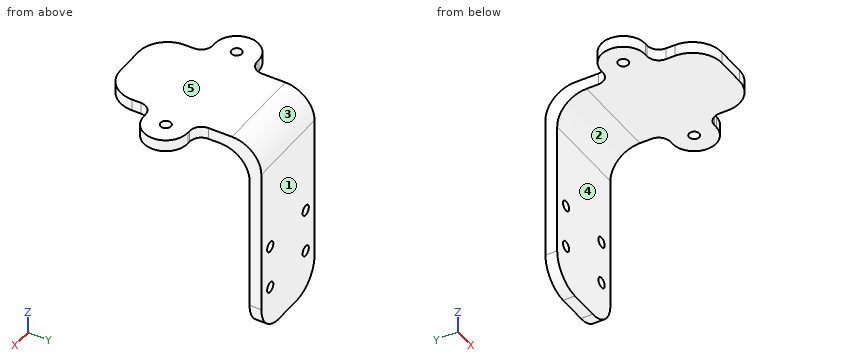
from build123d import *

# Parameters (mm, degrees)
SKETCH1_W            = 30
SKETCH1_H            = 70
BOSS_EXTRUDE1_DEPTH  = 2
SKETCH2_W            = 30
SKETCH2_H            = 4
BOSS_EXTRUDE2_DEPTH  = 50
SKETCH3_R            = 1.75
BOSS_EXTRUDE3_DEPTH  = 4
SKETCH4_R            = 1.75
CUT_EXTRUDE1_DEPTH   = 4
LPATTERN1_COUNT      = 2
LPATTERN1_PITCH      = 15
LPATTERN1_COUNT_DIR2 = 2
LPATTERN1_PITCH_DIR2 = 20
FILLET1_R            = 10
FILLET2_R            = 4


with BuildPart() as part:
    # Sketch1 → Boss-Extrude1 (new body, symmetric)
    with BuildSketch(Plane(origin=(0, 0, 0), x_dir=(1, 0, 0), z_dir=(0, 1, 0))):
        Rectangle(SKETCH1_W, SKETCH1_H)
    extrude(amount=BOSS_EXTRUDE1_DEPTH, both=True)

    # Sketch2 → Boss-Extrude2 (add)
    with BuildSketch(Plane.XZ.offset(2)):
        with Locations((0, 33)):
            Rectangle(SKETCH2_W, SKETCH2_H)
    extrude(amount=BOSS_EXTRUDE2_DEPTH)

    # Sketch3 → Boss-Extrude3 (add)
    with BuildSketch(Plane.XY.offset(35)):
        with BuildLine():
            Line((20, -20), (-20, -20))
            ThreePointArc((-20, -20), (-27.5, -27.5), (-20, -35))
            Line((-20, -35), (20, -35))
            ThreePointArc((20, -35), (27.5, -27.5), (20, -20))
        make_face()
        with Locations((-20, -27.5)):
            Circle(SKETCH3_R, mode=Mode.SUBTRACT)
        with Locations((20, -27.5)):
            Circle(SKETCH3_R, mode=Mode.SUBTRACT)
    extrude(amount=-BOSS_EXTRUDE3_DEPTH)

    # Sketch4 → Cut-Extrude1 (cut)
    with BuildSketch(Plane(origin=(0, 2, 0), x_dir=(1, 0, 0), z_dir=(0, 1, 0))):
        with Locations((-10, 20)):
            Circle(SKETCH4_R)
    cut_extrude1 = extrude(amount=-CUT_EXTRUDE1_DEPTH, mode=Mode.SUBTRACT)

    # LPattern1: Cut-Extrude1 2 × 2
    with Locations(*[(j * LPATTERN1_PITCH_DIR2, 0, i * LPATTERN1_PITCH) for i in range(LPATTERN1_COUNT) for j in range(LPATTERN1_COUNT_DIR2) if (i, j) != (0, 0)]):
        add(cut_extrude1, mode=Mode.SUBTRACT)

    # Fillet1
    fillet1_edges = [part.edges().sort_by_distance(p)[0] for p in [
        (0, -2, 31),
        (15, -52, 33),
        (0, 2, 35),
        (-15, -52, 33),
        (-15, 0, -35),
        (15, 0, -35),
    ]]
    fillet(fillet1_edges, radius=FILLET1_R)

    # Fillet2
    fillet2_edges = [part.edges().sort_by_distance(p)[0] for p in [
        (15, -35, 33),
        (-15, -35, 33),
        (15, -20, 33),
        (-15, -20, 33),
    ]]
    fillet(fillet2_edges, radius=FILLET2_R)


solid = part.part
Work out the finished part from the listing and answer in its coordinate system (mm). Face numbers are marked on the shaded views. A direction names the side the tool comes from. Give positions to 0.01 mm unless a question says otherwise; leave off trailing zeros. Loops run counter-clockwise (first coordinate to the right, second up) from the corner with the lowest first, then second, coordinate; pieces in that order, holes last. Notation, with made-up numbers: (45, -21.5) -> (65, -21.5) arc R32 ccw to (65, 9.5) -> close; hole circle Ø7 at (-34.75, 49.5). An arc over 180 degrees is marked (long way). Use a Markdown table: item, result. Add a question column.
1) Each of these flat-tipped pins is pushed along its axis until it touches: P1, Ø5, axis at x = 0, y = -25.5, coming from the -Z side; P2, Ø20, axis at y = -10.5, z = 3.5, coming from the +X side; P3, Ø1.1, axis at x = 19.5, z = 34, coming from the -Y side; P4, Ø6, axis at x = -17, z = 25, coming from the +Y side. Where does it stop, or does it pass through?
2) For a pull along Z with two mould halves and no side action, classify the marked faces 1, 2 and 3 as +Z half, -Z half, draft (parallel to the pull), parting line (faces both ways), or undercut.
3) The part is cut by section A-A, the plane y = -27.5. Determine the outline of the cut face in (x, z).
4) Which of the six approach directions +Z, -Z, +X, -X, +Y, -Y give full straight-line access (tool end or side, diameter ignored) to the marked faces 4 and 5?
5) The part is cut by section D-D, the plane x = -0.5. Determine the outline of the cut face in (y, z), plus the area to 3 significant figures.
6) The part is cut by section B-B, the plane z = -20. Determine the outline of the cut face in (x, y), plus the area to 3 significant figures.
7) Consider line 1 along X through (y, z) = (0, -5); line 2 along Z through (x, y) = (-10, 0); line 3 along Z through (x, y) = (-10, -0.85). Determine where each line is inside the solid, lowest interval first.
8) The part is cut by section C-C, the plane x = 10. Determine the outline of the cut face in (y, z), plus the area to 3 significant figures.
Reported:
| question | item | result |
|---|---|---|
| 1 | P1 | stops at z = 31 |
| 1 | P2 | stops at x = 15 |
| 1 | P3 | stops at y = -35 |
| 1 | P4 | stops at y = 2 |
| 2 | face 1 | draft |
| 2 | face 2 | -Z half |
| 2 | face 3 | +Z half |
| 3 | outline | (-27.5, 31) -> (-21.75, 31) -> (-21.75, 35) -> (-27.5, 35) -> close; (-18.25, 31) -> (18.25, 31) -> (18.25, 35) -> (-18.25, 35) -> close; (21.75, 31) -> (27.5, 31) -> (27.5, 35) -> (21.75, 35) -> close |
| 4 | face 4 | -Z, +X, -X, -Y |
| 4 | face 5 | +Z, +X, -X, +Y, -Y |
| 5 | outline | (-52, 31) -> (-12, 31) arc R10 cw to (-2, 21) -> (-2, -35) -> (2, -35) -> (2, 25) arc R10 ccw to (-8, 35) -> (-52, 35) -> close |
| 5 | area | 480 mm^2 |
| 6 | outline | (-15, -2) -> (-11.75, -2) -> (-11.75, 2) -> (-15, 2) -> close; (-8.25, -2) -> (8.25, -2) -> (8.25, 2) -> (-8.25, 2) -> close; (11.75, -2) -> (15, -2) -> (15, 2) -> (11.75, 2) -> close |
| 6 | area | 92.0 mm^2 |
| 7 | line 1 | x = -15 to -11.75, -8.25 to 8.25, 11.75 to 15 |
| 7 | line 2 | z = -33.66 to -21.75, -18.25 to -6.75, -3.25 to 31 |
| 7 | line 3 | z = -33.66 to -21.75, -18.25 to -6.75, -3.25 to 31.99 |
| 8 | outline | (-50.66, 31) -> (-12, 31) arc R10 cw to (-2, 21) -> (-2, -3.25) -> (2, -3.25) -> (2, 25) arc R10 ccw to (-8, 35) -> (-50.66, 35) -> close; (-2, -33.66) -> (2, -33.66) -> (2, -21.75) -> (-2, -21.75) -> close; (-2, -18.25) -> (2, -18.25) -> (2, -6.75) -> (-2, -6.75) -> close |
| 8 | area | 441 mm^2 |
